from build123d import *

# Parameters (mm, degrees)
BOSS_EXTRUDE1_DEPTH = 31.75
SKETCH3_W           = 12.7
SKETCH3_H           = 19.05
CUT_EXTRUDE1_DEPTH  = 6.35
SKETCH4_W           = 19.05
SKETCH4_H           = 6.35
CUT_EXTRUDE2_DEPTH  = 47.573244244


with BuildPart() as part:
    # Sketch2 → Boss-Extrude1 (new body)
    with BuildSketch(Plane.XY):
        Polygon((-18.228399123, 0), (26.221600877, 0), (26.221600877, 9.991502193), (-5.528399123, 9.991502193), (-5.528399123, 31.75), (-18.228399123, 31.75), align=None)
    extrude(amount=-BOSS_EXTRUDE1_DEPTH)

    # Sketch3 → Cut-Extrude1 (cut)
    with BuildSketch(Plane(origin=(0, 31.75, 0), x_dir=(1, 0, 0), z_dir=(0, 1, 0))):
        with Locations((-11.878399123, 15.875)):
            Rectangle(SKETCH3_W, SKETCH3_H)
    extrude(amount=-CUT_EXTRUDE1_DEPTH, mode=Mode.SUBTRACT)

    # Sketch4 → Cut-Extrude2 (cut, through all)
    with BuildSketch(Plane(origin=(0, 9.991502193, 0), x_dir=(1, 0, 0), z_dir=(0, 1, 0))):
        with Locations((16.696600877, 15.875)):
            Rectangle(SKETCH4_W, SKETCH4_H)
    extrude(amount=-CUT_EXTRUDE2_DEPTH, mode=Mode.SUBTRACT)


solid = part.part
Work out the finished part from the listing and answer in its coordinate system (mm). A direction names the side the tool comes from. Give positions to 0.01 mm unless a question says otherwise; leave off trailing zeros. Write each loop counter-clockwise with the first axis right and the second up, starting at its lowest first coordinate (ties: lowest second). Pieces come first, ordered by that corner, then holes.
Q1. The part is cut by section B-B on x = 22. Give the vertices of the cut face in (y, z), and give its area (3 significant figures).
Answer:
outline: (0, -31.75) - (9.99, -31.75) - (9.99, -19.05) - (0, -19.05) - close; (0, -12.7) - (9.99, -12.7) - (9.99, 0) - (0, 0) - close
area: 254 mm2
Q2. For a pull along Z with two mould halves and no side action, classify faces 6 (the face through (-1, 9, 0)), 7 (the face through (26.222, 5, -6)), 8 (the face through (17, 5, -12.7)), 9 (the face through (-12, 29, -25.4)) as released by +Z, released by -Z, zero draft, split by the parting line, or undercut.
Answer:
face 6: released by +Z
face 7: zero draft
face 8: undercut
face 9: undercut
Q3. The part is cut by section D-D on x = -10. Give the vertices of the cut face in (y, z).
Answer:
outline: (0, -31.75) - (31.75, -31.75) - (31.75, -25.4) - (25.4, -25.4) - (25.4, -6.35) - (31.75, -6.35) - (31.75, 0) - (0, 0) - close
Q4. The part is cut by section A-A on y = 28. Give the vertices of the cut face in (x, z), and give its area (3 significant figures).
Answer:
outline: (-18.23, -31.75) - (-5.53, -31.75) - (-5.53, -25.4) - (-18.23, -25.4) - close; (-18.23, -6.35) - (-5.53, -6.35) - (-5.53, 0) - (-18.23, 0) - close
area: 161 mm2
Q5. Straight lines are drawn through the part: L1, parallel to Y at x = 24, z = -26; L2, parallel to Z at x = -14.5, y = 27.5; L3, parallel to Z at x = 20, y = 5. For each, find the intervals that lie inside material, in ascending order.
Answer:
L1: y = 0 to 9.99
L2: z = -31.75 to -25.4, -6.35 to 0
L3: z = -31.75 to -19.05, -12.7 to 0
Q6. The part is cut by section C-C on z = -15.5. Give the vertices of the cut face in (x, y), and give its area (3 significant figures).
Answer:
outline: (-18.23, 0) - (7.17, 0) - (7.17, 9.99) - (-5.53, 9.99) - (-5.53, 25.4) - (-18.23, 25.4) - close
area: 449 mm2
Q7. Given pin 1 (9.5 mm diameter, centred on x = 16.5, z = -9.5, fed in from +Y); pin 2 (11 mm diameter, centred on y = 16, z = -12, fed in from +X); pin 3 (12 mm diameter, centred on x = 21.5, y = 19, fed in from +Z); pin 4 (4 mm diameter, centred on x = -14.5, z = -15.5, fed in from +Y), each flat-ended and moving along its own axis, determine where each tip first touches the part or whether it passes through.
Answer:
pin 1: stops at y = 9.99
pin 2: stops at x = -5.53
pin 3: passes through
pin 4: stops at y = 25.4
Q8. A tool of negligible diameter and unlimited length cuts with its end or side. For faces 1 (the face through (4, 0, -16)), 2 (the face through (-12, 25.4, -16)), 3 (the face through (7.172, 5, -16)), 4 (the face through (7, 9.992, -16)), 5 (the face through (26.222, 5, -25)), from which of +Z, -Z, +X, -X, +Y, -Y can it reach the whole face along a straight path? Write none if from no direction.
Answer:
face 1: +Z, -Z, +X, -X, -Y
face 2: +X, -X, +Y
face 3: +X, +Y, -Y
face 4: +Z, -Z, +X, +Y
face 5: +Z, -Z, +X, +Y, -Y
